```python
from build123d import *

# Parameters (mm, degrees)
F0_W     = 90
F0_H     = 44
F0_R     = 1.5
F0_W_2   = 70.5
F0_H_2   = 39
F1_DEPTH = 6.5
F3_DEPTH = 44.001
F4_SIZE  = 1
F6_R     = 2
F7_DEPTH = 90.001


with BuildPart() as f1:
    # F0 (on Top) → F1 (new body)
    with BuildSketch(Plane.XY):
        with Locations((18.801508, 8.04563)):
            Rectangle(F0_W, F0_H)
        with Locations((-21.698492, -10.45437)):
            Circle(F0_R, mode=Mode.SUBTRACT)
        with Locations((-20.198492, 8.04563)):
            Circle(F0_R, mode=Mode.SUBTRACT)
        with Locations((59.301508, -10.45437)):
            Circle(F0_R, mode=Mode.SUBTRACT)
        with Locations((57.801508, 8.04563)):
            Circle(F0_R, mode=Mode.SUBTRACT)
        with Locations((18.801508, 8.04563)):
            Rectangle(F0_W_2, F0_H_2, mode=Mode.SUBTRACT)
        with Locations((-21.698492, 26.54563)):
            Circle(F0_R, mode=Mode.SUBTRACT)
        with Locations((59.301508, 26.54563)):
            Circle(F0_R, mode=Mode.SUBTRACT)
    extrude(amount=F1_DEPTH)

    # F2 (on face) → F3 (cut, through all)
    with BuildSketch(Plane.XZ.offset(13.95437)):
        with BuildLine():
            ThreePointArc((63.801508, 0), (18.801508, 2.5), (-26.198492, 0))
            Line((-26.198492, 0), (63.801508, 0))
        make_face()
    extrude(amount=-F3_DEPTH, mode=Mode.SUBTRACT)

    # F4
    f4_edges = [f1.edges().sort_by_distance(p)[0] for p in [
        (57.801508, 26.54563, 6.5),
        (-23.198492, 26.54563, 6.5),
        (-23.198492, -10.45437, 6.5),
        (57.801508, -10.45437, 6.5),
    ]]
    chamfer(f4_edges, length=F4_SIZE)

    # F6
    f6_edges = [f1.edges().sort_by_distance(p)[0] for p in [
        (-16.448492, 27.54563, 3.733901),
        (54.051508, 27.54563, 3.733901),
        (54.051508, -11.45437, 3.733901),
        (-16.448492, -11.45437, 3.733901),
        (63.801508, 30.04563, 3.25),
        (63.801508, -13.95437, 3.25),
        (-26.198492, 30.04563, 3.25),
        (-26.198492, -13.95437, 3.25),
    ]]
    fillet(f6_edges, radius=F6_R)

    # F5 (on face) → F7 (cut, through all)
    with BuildSketch(Plane(origin=(-26.198492, 0, 0), x_dir=(0, -1, 0), z_dir=(-1, 0, 0))):
        Polygon((13.95437, 0), (-30.04563, 2.5), (-30.04563, 0), align=None)
    extrude(amount=-F7_DEPTH, mode=Mode.SUBTRACT)


solid = f1.part
```
Here's how the part is built. I have some questions about the finished solid (model axes, mm). A direction names the side the tool comes from. Coordinates: 2 decimals unless noted, no trailing zeros. Order: outer loops, then holes, each group sorted by start corner. A loop starts at its lowest first (then second) coordinate and runs counter-clockwise, first axis right, second up. Notation, with made-up numbers: M 56,9.5 L 78,9.5 A21 ccw 78,41.5 Z; hole C 71,-2 d2. An arc over 180 degrees is marked long. Answer as a JSON object with one key per item and string values. Group by question number.
(1) Suppose I cut it at C-C, the plane z = 4.5. Please give me the cut outline in (x, y).
(2) Suppose I cut it at A-A, the plane y = 16. Please give me the cut outline in (x, z), then the cut area to 3 significant figures.
(3) Which directions (+Z, -Z, +X, -X, +Y, -Y) give clear straight access to the entire face, cutting with the end or side of a thin tool? Please do faces 1 (the face through (18, 30.046, 4)), 2 (the face through (-15.88, 26.94, 4.4)).
(4) I need wall thicknesses on probe 1 along X at (y, z) = (2, 3); probe 2 along Y at (x, z) = (45.5, 6.25); probe 3 along X at (y, z) = (-10, 3). Which ranges of each line are inside material? Lowest first, please.
(5) If we mould it in two halves opening along X, with no side actions, what happens to faces 3 (the face through (-15.85, -10.88, 3.77)), 4 (the face through (63.802, 8, 4)), 5 (the face through (18, -11.454, 4)), 6 (the face through (18, -13.954, 4))? For each: released by +X, released by -X, zero draft, split by the parting line, or undercut.
(6) For pin 1 (3.5 mm diameter, centred on x = -21.7, y = 26.55, fed in from -Z); pin 2 (5 mm diameter, centred on x = -21.7, y = -10.45, fed in from -Z), each with a flat end and sliding along its axis, tell me the tip position at first contact or that it passes through.
(7) Suppose I cut it at B-B, the plane x = 1.5. Please give me the cut outline in (y, z), then the cut area to 3 significant figures.
Values found:
{
 "1": {"outline": "M -26.2,-11.95 A2 ccw -24.2,-13.95 L 61.8,-13.95 A2 ccw 63.8,-11.95 L 63.8,28.05 A2 ccw 61.8,30.05 L -24.2,30.05 A2 ccw -26.2,28.05 Z; hole C -21.7,-10.45 d3; hole C -21.7,26.55 d3; hole C -20.2,8.05 d3; hole M -16.45,-9.45 A2 ccw -14.45,-11.45 L 52.05,-11.45 A2 ccw 54.05,-9.45 L 54.05,25.55 A2 ccw 52.05,27.55 L -14.45,27.55 A2 ccw -16.45,25.55 Z; hole C 57.8,8.05 d3; hole C 59.3,-10.45 d3; hole C 59.3,26.55 d3"},
 "2": {"outline": "M -26.2,1.7 L -16.45,1.7 L -16.45,6.5 L -26.2,6.5 Z; M 54.05,1.7 L 63.8,1.7 L 63.8,6.5 L 54.05,6.5 Z", "area": "93.6 mm^2"},
 "3": {"face 1": "+Z, -Z, +X, -X, +Y", "face 2": "+Z, -Z"},
 "4": {"probe 1": "x = -26.2 to -16.45, 54.05 to 63.8", "probe 2": "y = -13.95 to -11.45, 27.55 to 30.05", "probe 3": "x = -26.2 to -23.13, -20.27 to -16.37, 53.98 to 57.87, 60.73 to 63.8"},
 "5": {"face 3": "undercut", "face 4": "released by +X", "face 5": "undercut", "face 6": "zero draft"},
 "6": {"pin 1": "stops at z = 2.2", "pin 2": "stops at z = 0.22"},
 "7": {"outline": "M -13.95,2.13 L -11.45,2.13 L -11.45,6.5 L -13.95,6.5 Z; M 27.55,2.36 L 30.05,2.5 L 30.05,6.5 L 27.55,6.5 Z", "area": "21.1 mm^2"}
}
